Here's how the part is built. I have some questions about the finished solid (model axes, mm). Face numbers are marked on the shaded views. A direction names the side the tool comes from. Coordinates: 2 decimals unless noted, no trailing zeros. Write each loop counter-clockwise with the first axis right and the second up, starting at its lowest first coordinate (ties: lowest second). Pieces come first, ordered by that corner, then holes.
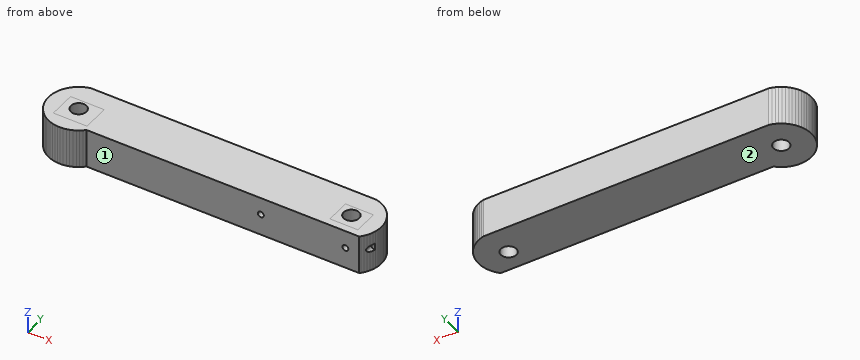
```python
from build123d import *
from OCP.BRepAlgoAPI import BRepAlgoAPI_Cut
from OCP.TopTools import TopTools_ListOfShape

# Parameters (mm, degrees)
BOSS_EXTRUDE1_DEPTH      = 19.999999553
CUT_EXTRUDE1_DEPTH       = 158.4379932
CUT_EXTRUDE2_DEPTH       = 158.4379932
SKETCH7_W                = 17.271465807
SKETCH7_H                = 13.849760317
SKETCH7_W_2              = 14.338575387
SKETCH7_H_2              = 12.546253463
BOSS_EXTRUDE4_DEPTH      = 20
SKETCH6_R                = 3.997536833
SKETCH6_R_2              = 3.982936498
CUT_EXTRUDE4_DEPTH       = 20
SPLIT1_SURFACE_1_BACK    = 175.651
SPLIT1_SURFACE_1_DEPTH   = 351.302
SPLIT1_SURFACE_2_BACK    = 175.651
SPLIT1_SURFACE_2_DEPTH   = 351.302
BODY_DELETE_KEEP_3_DEPTH = 19.999999553
SKETCH15_R               = 1.744345672
CUT_EXTRUDE8_DEPTH       = 6.604
SKETCH18_R               = 1.524
CUT_EXTRUDE10_DEPTH      = 6.604
SKETCH21_R               = 1.524
CUT_EXTRUDE12_DEPTH      = 6.604


with BuildPart() as part:
    # Sketch1 → Boss-Extrude1 (new body)
    with BuildSketch(Plane.XY.offset(19.999999553)):
        Polygon((-147.262692451, 13.588201255), (-148.526370525, 12.833039276), (-149.712219834, 11.960721575), (-150.809392333, 10.979211889), (-151.807874441, 9.897469543), (-152.69857645, 8.725371212), (-153.473347425, 7.473616395), (-154.125109315, 6.153633818), (-154.647916555, 4.777472466), (-155.037015676, 3.357697045), (-155.2888304, 1.907268073), (-155.401065946, 0.439427269), (-155.372709036, -1.032425207), (-155.203998089, -2.494852291), (-154.896497726, -3.934503533), (-154.453009367, -5.338235293), (-153.877556324, -6.69323327), (-153.175413609, -7.987127639), (-152.353018522, -9.208105505), (-151.417821646, -10.3450194), (-150.378391147, -11.387491599), (-149.244219065, -12.326003984), (-148.025646806, -13.15199025), (-146.733820438, -13.857908547), (-145.38051188, -14.437315054), (-143.978089094, -14.884918928), (-142.539337277, -15.196635388), (-141.077414155, -15.36961738), (-139.605656266, -15.402286313), (-138.137474656, -15.294345096), (-136.686325073, -15.046778135), (-135.265409946, -14.661843888), (-133.887723088, -14.143059961), (-132.565841079, -13.495159335), (-131.311833858, -12.724057771), (-130.137130618, -11.836796999), (-129.052475095, -10.841473937), (-10.947530158, -10.841473937), (-9.862869047, -11.836796999), (-8.688169532, -12.724057771), (-7.434152998, -13.495159335), (-6.112268195, -14.143059961), (-4.734582733, -14.661843888), (-3.313674591, -15.046778135), (-1.862514997, -15.294345096), (-0.394351926, -15.402286313), (1.077411231, -15.36961738), (2.539338311, -15.196635388), (3.978083376, -14.884918928), (5.380511284, -14.437315054), (6.733819377, -13.857908547), (8.025652729, -13.15199025), (9.244217537, -12.326003984), (10.378391482, -11.387491599), (11.417816393, -10.3450194), (12.35300675, -9.208105505), (13.175422326, -7.987127639), (13.877556659, -6.69323327), (14.453000389, -5.338235293), (14.896498062, -3.934503533), (15.204001218, -2.494852291), (15.372704715, -1.032425207), (15.401067212, 0.439427269), (15.288828872, 1.907268073), (15.03701508, 3.357697045), (14.647925273, 4.777472466), (14.125110582, 6.153633818), (13.473344967, 7.473616395), (12.698576786, 8.725371212), (11.807881296, 9.897469543), (10.809388012, 10.979211889), (9.71221365, 11.960721575), (8.526373655, 12.833039276), (7.262694649, 13.588201255), (5.932712927, 14.21931386), (4.548569676, 14.720613137), (3.122901777, 15.087526292), (-143.122896552, 15.087526292), (-144.548565149, 14.720613137), (-145.93270421, 14.21931386), align=None)
    extrude(amount=-BOSS_EXTRUDE1_DEPTH)

    # Sketch2 → Cut-Extrude1 (cut, through all)
    with BuildSketch(Plane(origin=(0, 0, 0), x_dir=(-1, 0, 0), z_dir=(0, 0, -1))):
        Polygon((138.905346394, 3.847302636), (138.217046857, 3.580653109), (137.589469552, 3.192068776), (137.043967843, 2.694782568), (136.599138379, 2.105728723), (136.270105839, 1.444966649), (136.068105698, 0.73499803), (136.000007391, 0), (136.068105698, -0.73499803), (136.270105839, -1.444966649), (136.599138379, -2.105728723), (137.043967843, -2.694782568), (137.589469552, -3.192068776), (138.217046857, -3.580653109), (138.905346394, -3.847302636), (139.630913734, -3.982936498), (140.369072556, -3.982936498), (141.094654799, -3.847302636), (141.782954335, -3.580653109), (142.41053164, -3.192068776), (142.956033349, -2.694782568), (143.400862813, -2.105728723), (143.729895353, -1.444966649), (143.931895494, -0.73499803), (143.999993801, 0), (143.931895494, 0.73499803), (143.729895353, 1.444966649), (143.400862813, 2.105728723), (142.956033349, 2.694782568), (142.41053164, 3.192068776), (141.782954335, 3.580653109), (141.094654799, 3.847302636), (140.369072556, 3.982936498), (139.630913734, 3.982936498), align=None)
    extrude(amount=-CUT_EXTRUDE1_DEPTH, mode=Mode.SUBTRACT)

    # Sketch3 → Cut-Extrude2 (cut, through all)
    with BuildSketch(Plane(origin=(0, 0, 0), x_dir=(-1, 0, 0), z_dir=(0, 0, -1))):
        Polygon((-2.956035547, 2.694782568), (-3.400868736, 2.105728723), (-3.729888937, 1.444966649), (-3.93189257, 0.73499803), (-4.00000019, 0), (-3.93189257, -0.73499803), (-3.729888937, -1.444966649), (-3.400868736, -2.105728723), (-2.956035547, -2.694782568), (-2.410538495, -3.192068776), (-1.78295339, -3.580653109), (-1.094651991, -3.847302636), (-0.369073445, -3.982936498), (0.369073445, -3.982936498), (1.094651991, -3.847302636), (1.78295339, -3.580653109), (2.410538495, -3.192068776), (2.956035547, -2.694782568), (3.400868736, -2.105728723), (3.729888937, -1.444966649), (3.93189257, -0.73499803), (4.00000019, 0), (3.93189257, 0.73499803), (3.729888937, 1.444966649), (3.400868736, 2.105728723), (2.956035547, 2.694782568), (2.410538495, 3.192068776), (1.78295339, 3.580653109), (1.094651991, 3.847302636), (0.369073445, 3.982936498), (-0.369073445, 3.982936498), (-1.094651991, 3.847302636), (-1.78295339, 3.580653109), (-2.410538495, 3.192068776), align=None)
    extrude(amount=-CUT_EXTRUDE2_DEPTH, mode=Mode.SUBTRACT)

    # Sketch7 → Boss-Extrude4 (add)
    with BuildSketch(Plane.XY):
        with Locations((-138.922924236, -1.542356043)):
            Rectangle(SKETCH7_W, SKETCH7_H)
        with Locations((0.715247426, -0.890602616)):
            Rectangle(SKETCH7_W_2, SKETCH7_H_2)
    extrude(amount=BOSS_EXTRUDE4_DEPTH)


with BuildPart() as cut_extrude4_tool:
    # Sketch6 → Cut-Extrude4 (new body)
    with BuildSketch(Plane.XY.offset(19.999999553)):
        with Locations((-139.974139817, 0.010018843)):
            Circle(SKETCH6_R)
        with Locations((-5.81e-07, 0)):
            Circle(SKETCH6_R_2)
    extrude(amount=-CUT_EXTRUDE4_DEPTH)


with BuildPart() as part_1:
    add(part.part)

    # Cut-Extrude4: cut by cut_extrude4_tool, with a tolerance
    cut_extrude4_stock = TopTools_ListOfShape()
    cut_extrude4_stock.Append(part_1.part.wrapped)
    cut_extrude4_tools = TopTools_ListOfShape()
    cut_extrude4_tools.Append(cut_extrude4_tool.part.wrapped)
    cut_extrude4_cut = BRepAlgoAPI_Cut()
    cut_extrude4_cut.SetArguments(cut_extrude4_stock)
    cut_extrude4_cut.SetTools(cut_extrude4_tools)
    cut_extrude4_cut.SetFuzzyValue(0.00001)
    cut_extrude4_cut.Build()
    add(Compound.cast(cut_extrude4_cut.Shape()).solids(), mode=Mode.REPLACE)


with BuildPart() as body_2:
    # Split1: the piece behind the surface
    add(part_1.part)
    # Split1 surface: a surface, the sketch's curves swept straight by 351.302 mm
    with BuildLine(Plane.XY.offset(-SPLIT1_SURFACE_1_BACK), mode=Mode.PRIVATE) as split1_surface_1_path:
        Line((-163.891257917, -10.841473937), (71.448565983, -10.841473937))
    split1_surface_1 = Shell.extrude(split1_surface_1_path.wire(), (0 * SPLIT1_SURFACE_1_DEPTH, 0 * SPLIT1_SURFACE_1_DEPTH, 1 * SPLIT1_SURFACE_1_DEPTH))
    split(bisect_by=split1_surface_1, keep=Keep.BOTTOM)

    # Body-Delete/Keep 3: read off the stored shape, not the designer's step
    # Body-Delete/Keep 3 outline → Body-Delete/Keep 3 (cut)
    with BuildSketch(Plane.XY):
        Polygon((10.92281306, -10.841473937), (-10.947530158, -10.841473937), (-9.862869047, -11.836796999), (-8.688169532, -12.724057771), (-7.434152998, -13.495159335), (-6.112268195, -14.143059961), (-4.734582733, -14.661843888), (-3.313674591, -15.046778135), (-1.862514997, -15.294345096), (-0.394351926, -15.402286313), (1.077411231, -15.36961738), (2.539338311, -15.196635388), (3.978083376, -14.884918928), (5.380511284, -14.437315054), (6.733819377, -13.857908547), (8.025652729, -13.15199025), (9.244217537, -12.326003984), (10.378391482, -11.387491599), align=None)
    extrude(amount=BODY_DELETE_KEEP_3_DEPTH, mode=Mode.SUBTRACT)


with BuildPart() as part_2:
    add(part_1.part)

    # Split1: split by a surface, the side it looks to stays
    # Split1 surface: a surface, the sketch's curves swept straight by 351.302 mm
    with BuildLine(Plane.XY.offset(-SPLIT1_SURFACE_2_BACK), mode=Mode.PRIVATE) as split1_surface_2_path:
        Line((-163.891257917, -10.841473937), (71.448565983, -10.841473937))
    split1_surface_2 = Shell.extrude(split1_surface_2_path.wire(), (0 * SPLIT1_SURFACE_2_DEPTH, 0 * SPLIT1_SURFACE_2_DEPTH, 1 * SPLIT1_SURFACE_2_DEPTH))
    split(bisect_by=split1_surface_2, keep=Keep.TOP)

    # Combine1: union body 2
    add(body_2.part)

    # Sketch15 → Cut-Extrude8 (cut)
    with BuildSketch(Plane(origin=(572.8274653, -10.841473937, -774.382334298), x_dir=(-1, 0, 0), z_dir=(0, -1, 0))):
        with Locations((558.238583002, -786.161559021)):
            Circle(SKETCH15_R)
    extrude(amount=-CUT_EXTRUDE8_DEPTH, mode=Mode.SUBTRACT)

    # Sketch18 → Cut-Extrude10 (cut)
    with BuildSketch(Plane(origin=(572.8274653, -10.841473937, -774.382334298), x_dir=(-1, 0, 0), z_dir=(0, -1, 0))):
        with Locations(Location((569.02222175, -785.202893663, 0), (0, 0, 90))):
            Circle(SKETCH18_R)
    extrude(amount=-CUT_EXTRUDE10_DEPTH, mode=Mode.SUBTRACT)

    # Sketch21 → Cut-Extrude12 (cut)
    with BuildSketch(Plane(origin=(572.8274653, -10.841473937, -774.382334298), x_dir=(-1, 0, 0), z_dir=(0, -1, 0))):
        with Locations(Location((612.380347085, -785.422094839, 0), (0, 0, 90))):
            Circle(SKETCH21_R)
    extrude(amount=-CUT_EXTRUDE12_DEPTH, mode=Mode.SUBTRACT)


solid = part_2.part
```
1) Imagine slicing it at B-B on x = -103.5. Please give me the cut outline in (y, z).
Values follow:
outline: (-10.84, 0) - (15.09, 0) - (15.09, 20) - (-10.84, 20) - close
2) I need wall thicknesses on probe 1 along X at (y, z) = (2.5, 5.75); probe 2 along Y at (x, z) = (0, 9.75); probe 3 along X at (y, z) = (3, 9). Which ranges of each line are inside material? Lowest first, please.
Values follow:
probe 1: x = -155.19 to -143.1, -136.85 to -3.1, 3.1 to 15.19
probe 2: y = -10.84 to -3.98, 3.98 to 15.09
probe 3: x = -155.1 to -142.63, -137.32 to -2.62, 2.62 to 15.1
3) Imagine slicing it at A-A on x = 0. Please give me the cut outline in (y, z).
Values follow:
outline: (-10.84, 0) - (-3.98, 0) - (-3.98, 20) - (-10.84, 20) - close; (3.98, 0) - (15.09, 0) - (15.09, 20) - (3.98, 20) - close
4) Will these pins go through, and if not, where does the flat tip stop? pin 1 (1.8 mm diameter, centred on x = -39.55, z = 11.04, fed in from -Y); pin 2 (5 mm diameter, centred on x = 0, y = 0, fed in from +Z); pin 3 (3.5 mm diameter, centred on x = -40, z = 11, fed in from -Y); pin 4 (8 mm diameter, centred on y = -3, z = 4.5, fed in from -X).
Values follow:
pin 1: stops at y = -4.24
pin 2: passes through
pin 3: stops at y = -10.84
pin 4: stops at x = -155.4
5) Imagine slicing it at C-C on z = 7.5. Count the separate pieces of the cut face and the enclosed holes in it, then the cut area to 3 significant figures.
Values follow:
separate pieces: 1
enclosed holes: 2
area: 4,270 mm2
6) On a 3-axis mill with a long thin cutter (end or side, diameter ignored), from which of +Z, -Z, +X, -X, +Y, -Y can I reach the whole of each face in a straight line? I mean the marked faces 1 and 2. Say none if no direction works.
Values follow:
face 1: +Z, -Z, +X, -Y
face 2: -Z, +X, -X, +Y, -Y
